Source: CAD feature listing. Evaluate the final solid. Frame: model axes, mm. Face numbers are marked on the shaded views. Coordinates: 2 decimals unless noted, no trailing zeros. One line per question, with ' | ' between items.
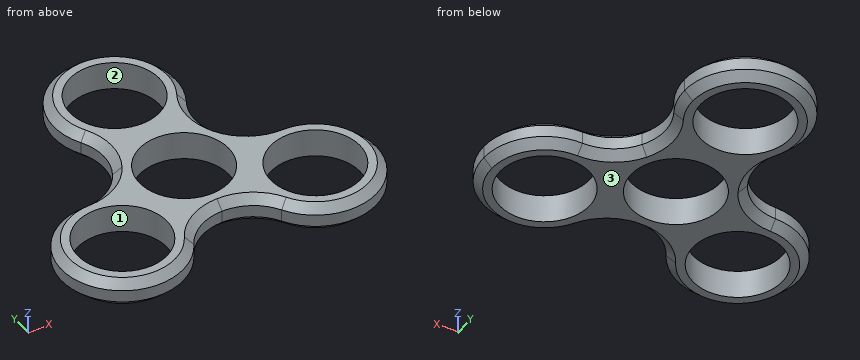
from build123d import *

# Parameters (mm, degrees)
F0_R     = 11
F1_DEPTH = 7
F2_R     = 12.499
F3_SIZE  = 2


# Not quite as in the source:
# - a fillet or chamfer is up to 0.001 mm smaller than in the source, because OpenCascade refuses the exact size


with BuildPart() as f1:
    # F0 (on Top) → F1 (new body)
    with BuildSketch(Plane.XY):
        with BuildLine():
            ThreePointArc((14.9052440041, -1.6833600857), (14.9762922658, -0.8430124372), (15, 0))
            ThreePointArc((15, 0), (12.5483433381, 8.2182163192), (5.9947894041, 13.75))
            ThreePointArc((5.9947894041, 13.75), (0, 12.5), (-5.9947894041, 13.75))
            ThreePointArc((-5.9947894041, 13.75), (-12.9903810568, 7.5), (-14.9052440041, -1.6833600857))
            ThreePointArc((-14.9052440041, -1.6833600857), (-10.8253175473, -6.25), (-8.9104546, -12.0666399143))
            ThreePointArc((-8.9104546, -12.0666399143), (0, -15), (8.9104546, -12.0666399143))
            ThreePointArc((8.9104546, -12.0666399143), (10.8253175473, -6.25), (14.9052440041, -1.6833600857))
        make_face()
        Circle(F0_R, mode=Mode.SUBTRACT)
        with BuildLine():
            ThreePointArc((-5.9947894041, 13.75), (0, 12.5), (5.9947894041, 13.75))
            ThreePointArc((5.9947894041, 13.75), (0, 15), (-5.9947894041, 13.75))
        make_face()
        with BuildLine():
            ThreePointArc((-5.9947894041, 13.75), (0, 15), (5.9947894041, 13.75))
            ThreePointArc((5.9947894041, 13.75), (12.5483433381, 19.2817836808), (15, 27.5))
            ThreePointArc((15, 27.5), (-8.2182163192, 40.0483433381), (-5.9947894041, 13.75))
        make_face()
        with Locations((0, 27.5)):
            Circle(F0_R, mode=Mode.SUBTRACT)
        with BuildLine():
            ThreePointArc((38.8156986041, -13.75), (30.5737745507, -0.3586442247), (14.9052440041, -1.6833600857))
            ThreePointArc((14.9052440041, -1.6833600857), (12.9903810568, -7.5), (8.9104546, -12.0666399143))
            ThreePointArc((8.9104546, -12.0666399143), (22.9726861669, -28.7262922658), (38.8156986041, -13.75))
        make_face()
        with Locations((23.8156986041, -13.75)):
            Circle(F0_R, mode=Mode.SUBTRACT)
        with BuildLine():
            ThreePointArc((8.9104546, -12.0666399143), (12.9903810568, -7.5), (14.9052440041, -1.6833600857))
            ThreePointArc((14.9052440041, -1.6833600857), (10.8253175473, -6.25), (8.9104546, -12.0666399143))
        make_face()
        with BuildLine():
            ThreePointArc((-8.9104546, -12.0666399143), (-10.8253175473, -6.25), (-14.9052440041, -1.6833600857))
            ThreePointArc((-14.9052440041, -1.6833600857), (-12.9903810568, -7.5), (-8.9104546, -12.0666399143))
        make_face()
        with BuildLine():
            ThreePointArc((-8.9104546, -12.0666399143), (-12.9903810568, -7.5), (-14.9052440041, -1.6833600857))
            ThreePointArc((-14.9052440041, -1.6833600857), (-37.2070543793, -20.5080759466), (-8.8156986041, -13.75))
            ThreePointArc((-8.8156986041, -13.75), (-8.8394063383, -12.9069875628), (-8.9104546, -12.0666399143))
        make_face()
        with Locations((-23.8156986041, -13.75)):
            Circle(F0_R, mode=Mode.SUBTRACT)
    extrude(amount=F1_DEPTH)

    # F2 (radius 12.5 in the source; OpenCascade refuses exactly that, so slightly less here)
    f2_edges = [f1.edges().sort_by_distance(p)[0] for p in [
        (-5.994789, 13.75, 3.5),
        (14.905244, -1.68336, 3.5),
        (-14.905244, -1.68336, 3.5),
        (5.994789, 13.75, 3.5),
        (-8.910455, -12.06664, 3.5),
        (8.910455, -12.06664, 3.5),
    ]]
    fillet(f2_edges, radius=F2_R)

    # F3
    f3_edges = [f1.edges().sort_by_distance(p)[0] for p in [
        (-6.250077, -16.674548, 0),
        (-6.250077, -16.674548, 7),
    ]]
    chamfer(f3_edges, length=F3_SIZE)


solid = f1.part
Item 1: Ray query, line 1 along Y through (x, z) = (0, 4.5); line 2 along Y through (x, z) = (0, 5.5); line 3 along X through (y, z) = (-20, 5.25). Return the intervals inside material, ascending. Write a range as [from, to].
Check sheet entries:
line 1: [-15, -11], [11, 16.5], [38.5, 42.5] | line 2: [-14.5, -11], [11, 16.5], [38.5, 42] | line 3: [-37.18, -32.87], [-14.76, -10.31], [10.31, 14.76], [32.87, 37.18]
Item 2: Mould query, pull axis X, two halves, no side actions, for the marked faces 1, 2 and 3. Classes: pulls with the +X half, pulls with the -X half, needs draft (parallel to the pull), parting line crosses it, or undercut.
Check sheet entries:
face 1: undercut | face 2: undercut | face 3: needs draft
Item 3: Pin query (flat end, axial travel): pin 1 Ø3 at (x, z) = (27.5, 2.5) entering from +Y; pin 2 Ø1.5 at (x, z) = (-7.5, 1) entering from +Y. Return the tip coordinate at first contact, or that it passes through.
Check sheet entries:
pin 1: y = 1.09 | pin 2: y = 40.3
Item 4: Cut plane A-A on y = -10. State how many separate pieces and enclosed holes the cut face has, and give its area (3 significant figures).
Check sheet entries:
separate pieces: 4 | enclosed holes: 0 | area: 175 mm²
